from build123d import *

# Parameters (mm, degrees)
F1_DEPTH    = 1.651
F2_R        = 6.0325
F3_DEPTH    = 8.89
F5_DEPTH    = 17.3228
F6_T2_ANGLE = 240.5568781665


# Not quite as in the source:
# - a fillet or chamfer that OpenCascade refuses, or shapes differently, is made with other operations: its cross-section is extruded or revolved along the edge and cut away or added


with BuildPart() as f1:
    # F0 (on Top) → F1 (new body)
    with BuildSketch(Plane.XY):
        with BuildLine():
            Line((-8.0826530047, 26.9640675335), (-8.0826530047, -6.4369324665))
            Line((-8.0826530047, -6.4369324665), (-11.0126939906, -23.0739324665))
            Line((-11.0126939906, -23.0739324665), (11.3393060094, -23.0739324665))
            Line((11.3393060094, -23.0739324665), (7.9193469953, -6.4369324665))
            Line((7.9193469953, -6.4369324665), (7.9193469953, 26.9640675335))
            ThreePointArc((7.9193469953, 26.9640675335), (-0.0816530047, 34.9650675335), (-8.0826530047, 26.9640675335))
        make_face()
    extrude(amount=F1_DEPTH)

    # F2 (on face) → F3 (join)
    with BuildSketch(Plane(origin=(0, 0, 0), x_dir=(1, 0, 0), z_dir=(0, 0, -1))):
        with Locations((-0.0816530047, -26.9640675335)):
            Circle(F2_R)
    extrude(amount=F3_DEPTH)

    # F4 (on face) → F5 (cut)
    with BuildSketch(Plane(origin=(-8.0826530047, 0, 0), x_dir=(0, -1, 0), z_dir=(-1, 0, 0))):
        Polygon((-24.261539802, -9.96281486), (-34.2662967741, -4.5080343261), (-34.2662967741, -10.2679394186), align=None)
    extrude(amount=-F5_DEPTH, mode=Mode.SUBTRACT)

    # F6: chamfer of 1.524 on 1 edges, made by hand

    # F6_s1 → F6_t2 (revolve, cut)
    with BuildSketch(Plane(origin=(-11.7615074362, 20.1448064433, 0), x_dir=(0, 0, 1), z_dir=(-0.5042026846, 0.8635853477, 0))):
        Polygon((-7.366, 19.5573408996), (-8.89, 18.0333408996), (-8.89, 19.5573408996), align=None)
    revolve(axis=Axis((-0.0816530047, 26.9640675335, -8.89), (0, 0, -1)), revolution_arc=F6_T2_ANGLE, mode=Mode.SUBTRACT)


solid = f1.part
CAD build for the part. Positions are in the model's coordinates, mm. A direction names the side the tool comes from. Coordinates: 2 decimals unless noted, no trailing zeros. Loops run counter-clockwise (first coordinate to the right, second up) from the corner with the lowest first, then second, coordinate; pieces in that order, holes last. Notation, with made-up numbers: (28, -34.5) - (37, -34.5) arc R34 ccw to (37, 2.5) - close; hole circle Ø6 at (-5, -34). An arc over 180 degrees is marked (long way). Write item = value, one per line. Start each with the question number.
Q1. Drill centre lines: L1, parallel to Z at x = 2.5, y = 4; L2, parallel to X at y = -5, z = 1.25; L3, parallel to Z at x = -4.5, y = 24. Where is each one in solid material? Low to high.
Q2. Cut at A-A, the plane y = 13. List the corners of the cut face in (x, z), then the cut area to 3 significant figures.
Q3. Cut at C-C, the plane z = -6. List the corners of the cut face in (x, y) (1 decimal).
Q4. Cut at B-B, the plane z = -2.75. List the corners of the cut face in (x, y) (1 decimal).
Q5. Which spindle directions (+Z, -Z, +X, -X, +Y, -Y) get a long thin tool onto all of the face, cutting with end or side? Do faces 1 (the flat face through (-8.083, 10, 1)), 2 (the flat face through (0, -23.074, 1)), 3 (the cylindrical face through (-1, 21, -4)), 4 (the flat face through (7.919, 10, 1)). Say none if no direction does.
Q6. Cut at D-D, the plane y = -17. List the corners of the cut face in (x, z), then the cut area to 3 significant figures.
Q7. Flat gauge pins, fed straight in: pin 1 Ø11 at (x, y) = (4.5, 15.5) entering from -Z; pin 2 Ø4 at (y, z) = (5, -1) entering from -X; pin 3 Ø5 at (y, z) = (27.5, -4.5) entering from +X; pin 4 Ø6 at (x, z) = (3, -0.5) entering from +Y. Where does each tip first touch, or does it go through?
Computed:
q1.L1 = 0 to 1.65
q1.L2 = -8.08 to 7.92
q1.L3 = -8.08 to 1.65
q2.outline = (-8.08, 0) - (7.92, 0) - (7.92, 1.65) - (-8.08, 1.65) - close
q2.area = 26.4 mm²
q3.outline = (-4, 31.5) arc R6 ccw (long way) to (3.9, 31.5) - close
q4.outline = circle Ø12.1 at (-0.1, 27)
q5.face_1 = +Z, -Z, -X, +Y
q5.face_2 = +Z, -Z, +X, -X, -Y
q5.face_3 = -Z
q5.face_4 = +Z, -Z, +X, +Y
q6.outline = (-9.94, 0) - (10.09, 0) - (10.09, 1.65) - (-9.94, 1.65) - close
q6.area = 33.1 mm²
q7.pin_1 = 0
q7.pin_2 = -8.08
q7.pin_3 = 5.95
q7.pin_4 = 34.96
